Model file for the job. Use its own axes, mm. Round coordinates to 2 decimals unless told otherwise and drop trailing zeros. Order: outer loops, then holes, each group sorted by start corner. A loop starts at its lowest first (then second) coordinate and runs counter-clockwise, first axis right, second up. Notation, with made-up numbers: M 0,57.25 L 22,57.25 A31 cw 22,85.25 Z; hole C -29,59 d1. An arc over 180 degrees is marked long. Return JSON: item names as keys, results as strings. Group by question number.
Item 1: Probe line 1 along X through (y, z) = (1.8, 0.5); line 2 along X through (y, z) = (-0.55, 0.3); line 3 along Z through (x, y) = (-4.5, -2.2). List the from-to ranges inside material, lowest first.
Item 2: Slice it at A-A on z = 0.25. Write the cut outline in (x, y).
Item 3: Pin check, flat tips, straight feed: pin 1 Ø0.8 at (x, y) = (-11.5, 0.5) entering from -Z; pin 2 Ø1 at (x, y) = (12, -2) entering from -Z. Stop position of each tip, or through.
from build123d import *

# Parameters (mm, degrees)
F0_W     = 29.8571444048
F0_H     = 6
F1_DEPTH = 1.38
F2_W     = 1
F2_H     = 6
F3_DEPTH = 0.76
F4_R     = 0.49999
F5_R     = 0.25


# Not quite as in the source:
# - a fillet or chamfer is up to 0.001 mm smaller than in the source, because OpenCascade refuses the exact size


with BuildPart() as f1:
    # F0 (on Top) → F1 (new body)
    with BuildSketch(Plane.XY):
        with Locations((2.9934216291, 0)):
            Rectangle(F0_W, F0_H)
    extrude(amount=F1_DEPTH)

    # F2 (on face) → F3 (cut)
    with BuildSketch(Plane(origin=(0, 0, 0), x_dir=(1, 0, 0), z_dir=(0, 0, -1))):
        with Locations((-11.4351505733, 0)):
            Rectangle(F2_W, F2_H)
        with Locations((-9.4351505733, 0)):
            Rectangle(F2_W, F2_H)
        with Locations((-7.4351505733, 0)):
            Rectangle(F2_W, F2_H)
        with Locations((-5.4351505733, 0)):
            Rectangle(F2_W, F2_H)
        with Locations((-3.4351505733, 0)):
            Rectangle(F2_W, F2_H)
    extrude(amount=-F3_DEPTH, mode=Mode.SUBTRACT)

    # F4 (radius 0.5 in the source; OpenCascade refuses exactly that, so slightly less here)
    f4_edges = [f1.edges().sort_by_distance(p)[0] for p in [
        (-10.935151, 0, 0),
        (-9.935151, 0, 0),
        (-8.935151, 0, 0),
        (-7.935151, 0, 0),
        (-6.935151, 0, 0),
        (-5.935151, 0, 0),
        (-4.935151, 0, 0),
        (-3.935151, 0, 0),
    ]]
    fillet(f4_edges, radius=F4_R)

    # F5
    f5_edges = [f1.edges().sort_by_distance(p)[0] for p in [
        (-10.935151, 0, 0.76),
        (-9.935151, 0, 0.76),
        (-8.935151, 0, 0.76),
        (-6.935151, 0, 0.76),
        (-4.935151, 0, 0.76),
        (-2.935151, 0, 0.76),
        (-3.935151, 0, 0.76),
        (-5.935151, 0, 0.76),
        (-7.935151, 0, 0.76),
    ]]
    fillet(f5_edges, radius=F5_R)


solid = f1.part
Output values:
{
 "1": {"line 1": "-10.94 to -9.94, -8.94 to -7.94, -6.94 to -5.94, -4.94 to -3.94, -2.94 to 17.92", "line 2": "-10.89 to -9.98, -8.89 to -7.98, -6.89 to -5.98, -4.89 to -3.98, -2.94 to 17.92", "line 3": "0 to 1.38"},
 "2": {"outline": "M -10.87,-3 L -10,-3 L -10,3 L -10.87,3 Z; M -8.87,-3 L -8,-3 L -8,3 L -8.87,3 Z; M -6.87,-3 L -6,-3 L -6,3 L -6.87,3 Z; M -4.87,-3 L -4,-3 L -4,3 L -4.87,3 Z; M -2.94,-3 L 17.92,-3 L 17.92,3 L -2.94,3 Z"},
 "3": {"pin 1": "z = 0.75", "pin 2": "z = 0"}
}
